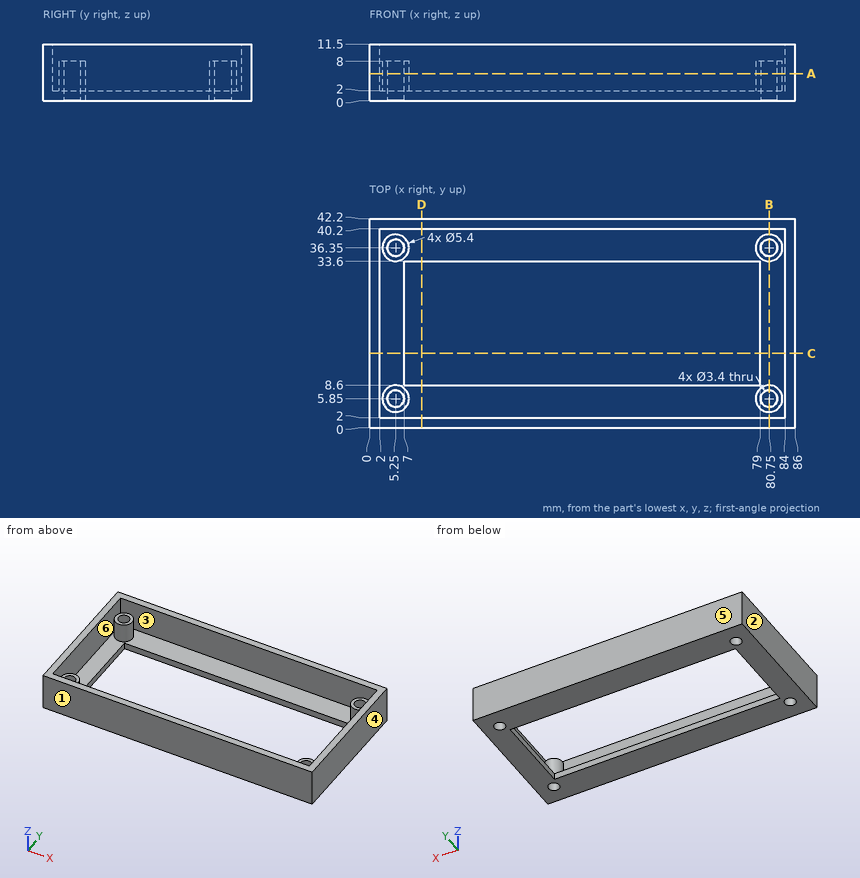
Job drawing, mm, ordinate dimensions from the low corner. One solid piece. A direction names the side the tool comes from. Round coordinates to 2 decimals unless told otherwise and drop trailing zeros. Order: outer loops, then holes, each group sorted by start corner. A loop starts at its lowest first (then second) coordinate and runs counter-clockwise, first axis right, second up. Notation, with made-up numbers: (-8, 47.5) - (4, 47.5) arc R23 ccw to (4, 63.5) - close; hole circle Ø4 at (5, 34.25). An arc over 180 degrees is marked (long way). Use CSV: the item, a comma, the result in double quotes. Start each with the question number.
1) Saw through at B-B (x = 80.75). List the corners of the cut face in (y, z).
2) Two-plate mould, pull along X, no slides. Class the marked faces 1, 2, 3 and 4: pulls with the +X half, pulls with the -X half, needs draft (parallel to the pull), parting line crosses it, or undercut.
3) Saw through at A-A (z = 5.5). Count the separate pieces of the cut face and the enclosed holes in it, and give its area (3 significant figures).
4) Pin check, flat tips, straight feed: pin 1 Ø1.6 at (x, y) = (80, 6) entering from +Z; pin 2 Ø4.5 at (x, y) = (5.5, 35.5) entering from +Z; pin 3 Ø19 at (x, y) = (51.5, 29.5) entering from +Z. Stop position of each tip, or through.
5) Tool access for the marked faces 5 and 6: list every direction of +Z, -Z, +X, -X, +Y, -Y with a clear straight run to the whole face (end or side of a thin tool).
6) Saw through at D-D (x = 10.5). List the corners of the cut face in (y, z), and give its area (3 significant figures).
7) Wall check: L1, parallel to Y at x = 80.75, z = 6; L2, parallel to Y at x = 48, z = 10.5; L3, parallel to X at y = 36, z = 0.5. Give the ranges that are in metal, low to high. Write a range as [from, to].
8) Saw through at C-C (y = 15). List the corners of the cut face in (x, z), and give its area (3 significant figures).
Values follow:
1,outline,"(0, 0) - (4.15, 0) - (4.15, 8) - (3.15, 8) - (3.15, 2) - (2, 2) - (2, 11.5) - (0, 11.5) - close; (7.55, 0) - (34.65, 0) - (34.65, 8) - (33.65, 8) - (33.65, 2) - (8.55, 2) - (8.55, 8) - (7.55, 8) - close; (38.05, 0) - (42.2, 0) - (42.2, 11.5) - (40.2, 11.5) - (40.2, 2) - (39.05, 2) - (39.05, 8) - (38.05, 8) - close"
2,face 1,"needs draft"
2,face 2,"pulls with the -X half"
2,face 3,"undercut"
2,face 4,"pulls with the +X half"
3,separate pieces,"5"
3,enclosed holes,"5"
3,area,"552 mm2"
4,pin 1,"passes through"
4,pin 2,"stops at z = 8"
4,pin 3,"stops at z = 2"
5,face 5,"+Z, -Z, +X, -X, +Y"
5,face 6,"+Z"
6,outline,"(0, 0) - (8.6, 0) - (8.6, 2) - (2, 2) - (2, 11.5) - (0, 11.5) - close; (33.6, 0) - (42.2, 0) - (42.2, 11.5) - (40.2, 11.5) - (40.2, 2) - (33.6, 2) - close"
6,area,"72.4 mm2"
7,L1,"y = [0, 2], [3.15, 4.15], [7.55, 8.55], [33.65, 34.65], [38.05, 39.05], [40.2, 42.2]"
7,L2,"y = [0, 2], [40.2, 42.2]"
7,L3,"x = [0, 3.59], [6.91, 79.09], [82.41, 86]"
8,outline,"(0, 0) - (7, 0) - (7, 2) - (2, 2) - (2, 11.5) - (0, 11.5) - close; (79, 0) - (86, 0) - (86, 11.5) - (84, 11.5) - (84, 2) - (79, 2) - close"
8,area,"66.0 mm2"
